from build123d import *

# Parameters (mm, degrees)
BOSS_EXTRUDE1_DEPTH = 59.999999888
CUT_EXTRUDE1_START  = 60
CUT_EXTRUDE1_DEPTH  = 53.65
SKETCH4_R           = 1.700000029
CUT_EXTRUDE2_DEPTH  = 7.35


with BuildPart() as part:
    # Sketch1 → Boss-Extrude1 (new body)
    with BuildSketch(Plane(origin=(0, 0, 0), x_dir=(1, 0, 0), z_dir=(0, 1, 0))):
        with BuildLine():
            Line((50.8, 79.121), (0, 79.121))
            Line((0, 79.121), (0, 0))
            Line((0, 0), (57.15, 0))
            ThreePointArc((57.15, 0), (47.890801483, 39.072201564), (50.8, 79.121))
        make_face()
    extrude(amount=BOSS_EXTRUDE1_DEPTH)

    # Sketch3 → Cut-Extrude1 (cut)
    with BuildSketch(Plane(origin=(0, 0, 0), x_dir=(1, 0, 0), z_dir=(0, 1, 0)).offset(CUT_EXTRUDE1_START)):
        with BuildLine():
            Line((51.265506183, -2.386468628), (0, 0))
            Line((0, 0), (0, 79.121))
            Line((0, 79.121), (44.293451527, 79.121))
            ThreePointArc((44.293451527, 79.121), (41.621147879, 37.840489172), (51.265506183, -2.386468628))
        make_face()
    extrude(amount=-CUT_EXTRUDE1_DEPTH, mode=Mode.SUBTRACT)

    # Sketch4 → Cut-Extrude2 (cut, through all)
    with BuildSketch(Plane(origin=(0, 6.35, 0), x_dir=(1, 0, 0), z_dir=(0, 1, 0))):
        with Locations((6.35, 72.771)):
            Circle(SKETCH4_R)
        with Locations((25.4, 72.771)):
            Circle(SKETCH4_R)
        with Locations((6.35, 9.271)):
            Circle(SKETCH4_R)
    extrude(amount=-CUT_EXTRUDE2_DEPTH, mode=Mode.SUBTRACT)


solid = part.part
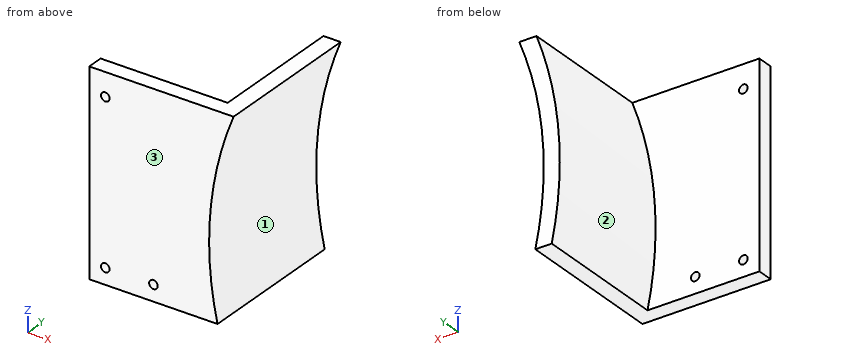
Design review of the part built by this model. Coordinates are the model's own, in mm. Face numbers are marked on the shaded views. Give positions to 0.01 mm unless a question says otherwise; leave off trailing zeros. Loops run counter-clockwise (first coordinate to the right, second up) from the corner with the lowest first, then second, coordinate; pieces in that order, holes last. Notation, with made-up numbers: (-3, 50.5) - (40, 50.5) arc R28 ccw to (40, 75.5) - close; hole circle Ø9 at (45, 61.25). An arc over 180 degrees is marked (long way). Use CSV: the item, a comma, the result in double quotes. Start each with the question number.
1. Add section B-B (x = 25.4). State the section outline as (y, z) points, plus the area to 3 significant figures.
2. Add section A-A (x = 6.35). State the section outline as (y, z) points, plus the area to 3 significant figures.
3. Wall thickness on L1, parallel to Z at x = 6.35, y = 1.75; L2, parallel to Z at x = 6, y = 4; L3, parallel to Y at x = 41.5, z = -37: over which ranges is each line inside the solid? List them lowest first.
4. Draft analysis for pull direction Z (two halves, no side actions). For the marked faces 1, 2 and 3, state which applies: released by +Z, released by -Z, zero draft, split by the parting line, or undercut.
5. Add section C-C (z = -63.5). State the section outline as (x, y) points.
6. Insertion check: P1, Ø4.5, axis at x = 6.35, z = -72.771, coming from the -Y side; P2, Ø1.5, axis at x = 25.5, z = -25, coming from the +Y side; P3, Ø1, axis at y = 23.5, z = -61, coming from the +X side. Each pin has a flat end and moves straight along its axis. Give the tip position at first contact, or say it passes through.
7. Add section D-D (y = 28). State the section outline as (x, z) points.
Results found:
1,outline,"(0, -79.12) - (6.35, -79.12) - (6.35, -74.47) - (0, -74.47) - close; (0, -71.07) - (6.35, -71.07) - (6.35, 0) - (0, 0) - close"
1,area,"481 mm²"
2,outline,"(0, -79.12) - (6.35, -79.12) - (6.35, -74.47) - (0, -74.47) - close; (0, -71.07) - (6.35, -71.07) - (6.35, -10.97) - (0, -10.97) - close; (0, -7.57) - (6.35, -7.57) - (6.35, 0) - (0, 0) - close"
2,area,"459 mm²"
3,L1,"z = -79.12 to -74.47, -71.07 to -10.97, -7.57 to 0"
3,L2,"z = -79.12 to -74.43, -71.11 to -10.93, -7.61 to 0"
3,L3,"y = 0 to 6.35"
4,face 1,"undercut"
4,face 2,"split by the parting line"
4,face 3,"zero draft"
5,outline,"(0, 0) - (48.2, 0) - (48.2, 60) - (41.81, 60) - (41.81, 6.35) - (0, 6.35) - close"
6,P1,"stops at y = 0"
6,P2,"stops at y = 6.35"
6,P3,"stops at x = 48"
7,outline,"(44.29, -79.12) - (50.8, -79.12) arc R132.08 cw to (57.15, 0) - (50.32, 0) arc R138.43 ccw to start"
